from build123d import *

# Parameters (mm, degrees)
EXTRUDE_1_DEPTH              = 6
HOLE_WIZARD_M5_1_D           = 8
HOLE_WIZARD_M5_1_CBORE_D     = 9.5
HOLE_WIZARD_M5_1_CBORE_DEPTH = 0.9
SKETCH_7_R                   = 1.5
CUT_EXTRUDE_1_DEPTH          = 1
CUT_EXTRUDE_1_DEPTH_BACK     = 7


with BuildPart() as part:
    # 草图1 → 凸台-拉伸1 (new body)
    with BuildSketch(Plane.XY):
        with BuildLine():
            Line((-60, -10), (135, -10))
            ThreePointArc((135, -10), (145, 0), (135, 10))
            Line((135, 10), (6, 10))
            Line((6, 10), (6, 15))
            ThreePointArc((6, 15), (0, 21), (-6, 15))
            Line((-6, 15), (-6, 10))
            Line((-6, 10), (-60, 10))
            ThreePointArc((-60, 10), (-70, 0), (-60, -10))
        make_face()
    extrude(amount=EXTRUDE_1_DEPTH)

    # M5 六角头螺栓的柱形沉头孔1 (through all)
    with Locations(Plane(origin=(0, 0, 6), x_dir=(-1, 0, 0), z_dir=(0, 0, 1))):
        with Locations((-135, 0), (60, 0), (0, 0)):
            CounterBoreHole(HOLE_WIZARD_M5_1_D / 2, HOLE_WIZARD_M5_1_CBORE_D / 2, HOLE_WIZARD_M5_1_CBORE_DEPTH)

    # 草图7 → 切除-拉伸1 (cut, two sides)
    with BuildSketch(Plane(origin=(0, 0, 0), x_dir=(-1, 0, 0), z_dir=(0, 0, -1))) as cut_extrude_1_sk:
        with Locations((-37.5, 0)):
            Circle(SKETCH_7_R)
        with Locations((-90, 0)):
            Circle(SKETCH_7_R)
        with Locations((32, 0)):
            Circle(SKETCH_7_R)
        with Locations((0, 15)):
            Circle(SKETCH_7_R)
    extrude(amount=CUT_EXTRUDE_1_DEPTH, mode=Mode.SUBTRACT)
    extrude(cut_extrude_1_sk.sketch, amount=-CUT_EXTRUDE_1_DEPTH_BACK, mode=Mode.SUBTRACT)


solid = part.part
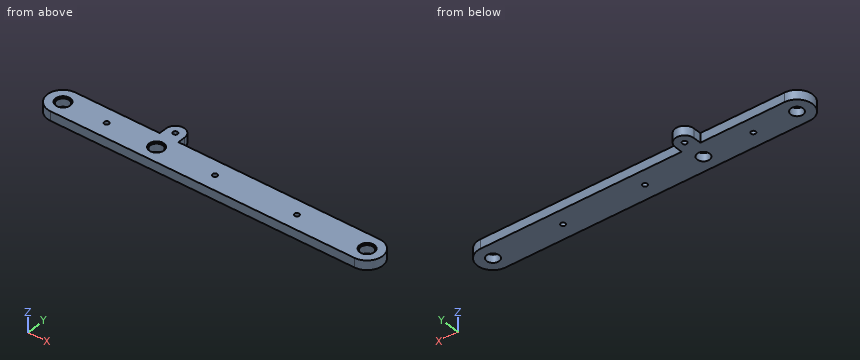
Can you work these out from the model? Positions are in its coordinate system, mm. Coordinates: 2 decimals unless noted, no trailing zeros. Loops run counter-clockwise (first coordinate to the right, second up) from the corner with the lowest first, then second, coordinate; pieces in that order, holes last. Notation, with made-up numbers: (72.5, 43) - (105.5, 43) arc R29 ccw to (105.5, 69) - close; hole circle Ø2 at (-8, -26). An arc over 180 degrees is marked (long way). Answer as a JSON object with one key per item and string values. Group by question number.
Item 1: If I drill on L1, parallel to Y at x = 37.5, z = 4.75; L2, parallel to Y at x = -60, z = 5.4; L3, parallel to Y at x = 94.5, z = 5.45, over which ranges is the centre line in solid material (lowest first)? Write a range as from..to.
Item 2: If we section it at A-A (z = 2.6): List the corners of the cut face in (x, y) for me, plus the area to 3 significant figures.
Item 3: If we section it at C-C (y = 6.5): List the corners of the cut face in (x, z) for me.
Item 4: If we section it at B-B (x = -45.5): List the corners of the cut face in (y, z) for me, plus the area to 3 significant figures.
Item 5: For pin 1 (1.8 mm diameter, centred on x = 49, z = 4, fed in from +Y); pin 2 (1.5 mm diameter, centred on y = 12, z = 3, fed in from -X), each with a flat end and sliding along its axis, tell me the tip position at first contact or that it passes through.
Returned:
{
 "1": {"L1": "y = -10..-1.5, 1.5..10", "L2": "y = -10..-4.75, 4.75..10", "L3": "y = -10..10"},
 "2": {"outline": "(-60, -10) - (135, -10) arc R10 ccw to (135, 10) - (6, 10) - (6, 15) arc R6 ccw to (-6, 15) - (-6, 10) - (-60, 10) arc R10 ccw to start; hole circle Ø8 at (-60, 0); hole circle Ø3 at (-32, 0); hole circle Ø8 at (0, 0); hole circle Ø3 at (0, 15); hole circle Ø3 at (37.5, 0); hole circle Ø3 at (90, 0); hole circle Ø8 at (135, 0)", "area": "4,150 mm²"},
 "3": {"outline": "(-67.6, 0) - (142.6, 0) - (142.6, 6) - (-67.6, 6) - close"},
 "4": {"outline": "(-10, 0) - (10, 0) - (10, 6) - (-10, 6) - close", "area": "120 mm²"},
 "5": {"pin 1": "stops at y = 10", "pin 2": "stops at x = -6"}
}
